Source: CAD feature listing. Evaluate the final solid. Frame: model axes, mm. Face numbers are marked on the shaded views. A direction names the side the tool comes from. Coordinates: 2 decimals unless noted, no trailing zeros. Write each loop counter-clockwise with the first axis right and the second up, starting at its lowest first coordinate (ties: lowest second). Pieces come first, ordered by that corner, then holes. Notation, with made-up numbers: M 0.25,16 L 6.25,16 A32 ccw 6.25,52 Z; hole C 87.25,21.25 d1. An arc over 180 degrees is marked long. Answer as CSV lines item,"result". Start each with the question number.
1. Contact query for flat-ended pins moving along their axis: pin 1 Ø4 at (y, z) = (3, -8.5) entering from -X; pin 2 Ø1.5 at (y, z) = (-1, -36) entering from +X; pin 3 Ø1 at (x, y) = (2.5, -1) entering from -Z. Output: stop coordinate, or through.
2. Section A-A on x = 0. Return the cut outline in (y, z) (3 decimals).
3. Section B-B on z = -19.5. Return the cut outline in (x, y), plus the area to 3 significant figures.
4. Reachability of the marked faces 1 and 2 from +Z, -Z, +X, -X, +Y, -Y: full face, straight path, thin tool, end or side. Return the list, or none.
5. Line query: probe 1 along Z at (x, y) = (-1, 0); probe 2 along Z at (x, y) = (3, 1); probe 3 along Y at (x, z) = (0.25, -53). Output: solid intervals per line, ascending. Write a range as [from, to].
Autodesk Inventor part; units mm, degrees
ref_plane "YZ Plane" through (0, 0, 0) normal (1, 0, 0) x (0, 1, 0)
ref_plane "XZ Plane" through (0, 0, 0) normal (0, 1, 0) x (-1, 0, 0)
ref_plane "XY Plane" through (0, 0, 0) normal (0, 0, 1) x (1, 0, 0)
sketch "Sketch1" plane through (0, 0, 0) normal (0, 0, 1) x (1, 0, 0)
  circle A0 centre (0, 0) radius 3.9624
  dimension "d0" = 7.9248
extrude "Extrusion1" add sketch "Sketch1" along normal blind 4.826
sketch "Sketch2" plane through (0, 0, 0) normal (0, 0, -1) x (-1, 0, 0)
  circle A0 centre (0, 0) radius 3.9624
  circle A1 centre (0, 0) radius 2.413
  dimension "d3" = 4.826
extrude "Extrusion2" add sketch "Sketch2" along normal blind 57.15 contours A1
sketch "Sketch3" plane through (0, 0, 4.826) normal (0, 0, 1) x (1, 0, 0)
  circle A0 centre (0, 0) radius 3.9624
  line L0 (-1.1457, 1.9844) -> (1.1457, 1.9844)
  line L1 (1.1457, 1.9844) -> (2.2914, 0)
  line L2 (2.2914, 0) -> (1.1457, -1.9844)
  line L3 (1.1457, -1.9844) -> (-1.1457, -1.9844)
  line L4 (-1.1457, -1.9844) -> (-2.2914, 0)
  line L5 (-2.2914, 0) -> (-1.1457, 1.9844)
  dimension "d6" = 3.9688
extrude "Extrusion3" cut sketch "Sketch3" against normal blind 3.175 contours L0 L1 L2 L3 L4 L5
thread "Thread1"
chamfer "Chamfer1" distance 0.508 angle 45 1 edges at (2.413, 0, -57.15)
chamfer "Chamfer2" distance 0.508 angle 45 1 edges at (-3.9624, 0, 4.826)
properties part number "10-32 x1000" material "Steel"
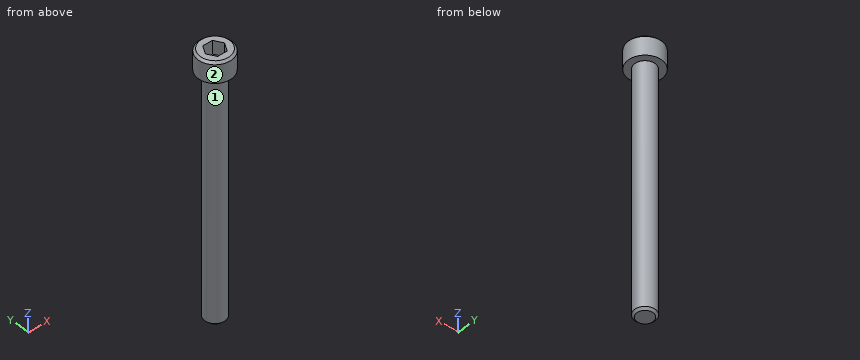
Values:
1,pin 1,"x = -2.2"
1,pin 2,"x = 2.4"
1,pin 3,"z = -56.86"
2,outline,"M -3.962,0 L -2.413,0 L -2.413,-56.642 L -1.905,-57.15 L 1.905,-57.15 L 2.413,-56.642 L 2.413,0 L 3.962,0 L 3.962,4.318 L 3.454,4.826 L 1.984,4.826 L 1.984,1.651 L -1.984,1.651 L -1.984,4.826 L -3.454,4.826 L -3.962,4.318 Z"
3,outline,"C 0,0 d4.83"
3,area,"18.3 mm²"
4,face 1,"-Z"
4,face 2,"+Z, -Z"
5,probe 1,"[-57.15, 1.65]"
5,probe 2,"[0, 4.83]"
5,probe 3,"[-2.4, 2.4]"
